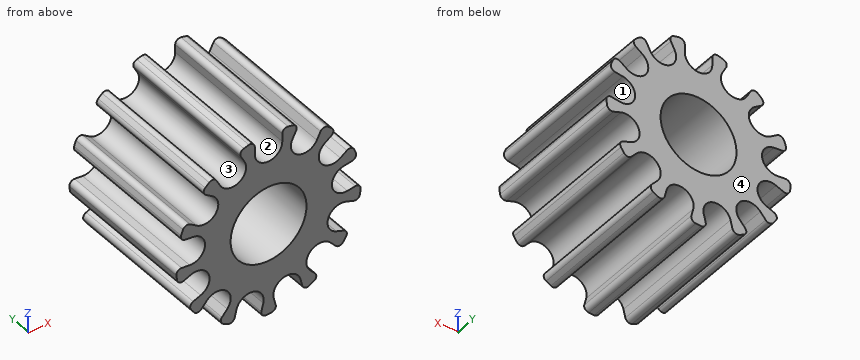
from build123d import *

# Parameters (mm, degrees)
BOSS_EXTRUDE1_DEPTH      = 7.5
CUT_EXTRUDE1_START       = -7.5
CUT_EXTRUDE1_DEPTH       = 15
FILLET1_R                = 0.5
CIRPATTERN1_COUNT        = 13
FILLET1_OF_CIRPATTERN1_R = 0.5
CUT_EXTRUDE2_DEPTH       = 16.666124697
CUT_EXTRUDE2_DEPTH_BACK  = 16.666124697
SKETCH7_R                = 4


# Read off the part's stored shape, not the designer's step: Cut-Extrude1
with BuildPart() as part:
    # Sketch5 → Boss-Extrude1 (new, symmetric)
    with BuildSketch(Plane(origin=(0, 0, 0), x_dir=(1, 0, 0), z_dir=(0, 1, 0))):
        with BuildLine():
            ThreePointArc((-0.898321896, 9.703578331), (-2.332148212, 9.46189724), (-3.714053167, 9.009562905))
            Line((-3.714053167, 9.009562905), (-3.369074568, 7.60992971))
            ThreePointArc((-3.369074568, 7.60992971), (-1.614201219, 6.549071788), (-0.553343297, 8.303945136))
            Line((-0.553343297, 8.303945136), (-0.898321896, 9.703578331))
        make_face()
        with BuildLine():
            Line((-3.369074568, 7.60992971), (-3.714053167, 9.009562905))
            ThreePointArc((-3.714053167, 9.009562905), (-5.420917899, -8.098151875), (9.745071301, 0))
            ThreePointArc((9.745071301, 0), (6.565523731, 7.201410473), (-0.898321896, 9.703578331))
            Line((-0.898321896, 9.703578331), (-0.553343297, 8.303945136))
            ThreePointArc((-0.553343297, 8.303945136), (-1.614201219, 6.549071788), (-3.369074568, 7.60992971))
        make_face()
    extrude(amount=BOSS_EXTRUDE1_DEPTH, both=True)

    # Cut-Extrude1 outline → Cut-Extrude1 (cut)
    with BuildSketch(Plane(origin=(0, 0, 0), x_dir=(1, 0, 0), z_dir=(0, 1, 0)).offset(CUT_EXTRUDE1_START)):
        with BuildLine():
            ThreePointArc((-0.898321896, 9.703578331), (-2.332148212, 9.46189724), (-3.714053167, 9.009562905))
            Line((-3.714053167, 9.009562905), (-3.369074568, 7.60992971))
            ThreePointArc((-3.369074568, 7.60992971), (-1.61420122, 6.549071788), (-0.553343297, 8.303945136))
            Line((-0.553343297, 8.303945136), (-0.898321896, 9.703578331))
        make_face()
    cut_extrude1 = extrude(amount=CUT_EXTRUDE1_DEPTH, mode=Mode.SUBTRACT)

    # Fillet1
    fillet1_edges = [part.edges().sort_by_distance(p)[0] for p in [
        (-3.714053167, 0, -9.009562905),
        (-0.898321896, 0, -9.703578331),
    ]]
    fillet(fillet1_edges, radius=FILLET1_R)

    # CirPattern1: Cut-Extrude1 ×13 about axis
    cirpattern1_axis = Axis((0, 0, 0), (0, 1, 0))
    for i in range(1, CIRPATTERN1_COUNT):
        add(cut_extrude1.rotate(cirpattern1_axis, i * 360 / CIRPATTERN1_COUNT), mode=Mode.SUBTRACT)

    # Fillet1 of CirPattern1
    fillet1_of_cirpattern1_edges = [part.edges().sort_by_distance(p)[0] for p in [
        (-7.475583408, 0, -6.251565194),
        (-5.304902238, 0, -8.174620903),
        (-9.524547581, 0, -2.061409236),
        (-8.496193408, 0, -4.77295634),
        (-9.391552687, 0, 2.600990735),
        (-9.741109059, 0, -0.277865001),
        (-7.107066252, 0, 6.667535074),
        (-8.754454018, 0, 4.280881862),
        (-3.194436588, 0, 9.20662748),
        (-5.762259063, 0, 7.85893028),
        (1.45, 0, 9.636592482),
        (-1.45, 0, 9.636592482),
        (5.762259064, 0, 7.85893028),
        (3.194436589, 0, 9.206627479),
        (8.754454018, 0, 4.280881862),
        (7.107066252, 0, 6.667535073),
        (9.741109059, 0, -0.277865001),
        (9.391552686, 0, 2.600990734),
        (8.496193408, 0, -4.772956341),
        (9.524547581, 0, -2.061409237),
        (5.304902238, 0, -8.174620903),
        (7.475583408, 0, -6.251565194),
        (0.898321896, 0, -9.703578332),
        (3.714053167, 0, -9.009562905),
    ]]
    fillet(fillet1_of_cirpattern1_edges, radius=FILLET1_OF_CIRPATTERN1_R)

    # Sketch7 → Cut-Extrude2 (cut, two sides: drawn at the far end of the back side and taken through both)
    with BuildSketch(Plane(origin=(0, 0, 0), x_dir=(1, 0, 0), z_dir=(0, 1, 0)).offset(-CUT_EXTRUDE2_DEPTH_BACK)):
        with Locations(Location((0, 0, 0), (0, 0, 270))):
            Circle(SKETCH7_R)
    extrude(amount=CUT_EXTRUDE2_DEPTH + CUT_EXTRUDE2_DEPTH_BACK, mode=Mode.SUBTRACT)


solid = part.part
The model under review builds one solid part; all positions refer to its coordinate system, in mm. Face numbers are marked on the shaded views. A direction names the side the tool comes from. Coordinates: 2 decimals unless noted, no trailing zeros. Write each loop counter-clockwise with the first axis right and the second up, starting at its lowest first coordinate (ties: lowest second). Pieces come first, ordered by that corner, then holes. Notation, with made-up numbers: (26, -30.5) -> (62, -30.5) arc R14 cw to (62, -23.5) -> close; hole circle Ø6 at (40.25, 62.25). An arc over 180 degrees is marked (long way). Answer in a Markdown table with one row per item.
1. Draft analysis for pull direction X (two halves, no side actions). For the marked faces 3 and 4, state which applies: +X half, -X half, draft (parallel to the pull), parting line (faces both ways), or undercut.
Answers below:
| item | result |
|---|---|
| face 3 | undercut |
| face 4 | draft |
2. For the marked faces 1 and 2, list the 3-axis set-ups (+Z, -Z, +X, -X, +Y, -Y) from which the entire face can be reached by the end or side of a thin tool; tool diameter is ignored.
Answers below:
| item | result |
|---|---|
| face 1 | +Y, -Y |
| face 2 | +Z, +Y, -Y |
3. Wall thickness on probe 1 along X at (y, z) = (0, 0); probe 2 along Z at (x, y) = (0, -0.5); probe 3 along X at (y, z) = (6.5, 6): over which ranges is each line inside the solid? List them lowest first. Write a range as [from, to].
Answers below:
| item | result |
|---|---|
| probe 1 | x = [-7.07, -4], [4, 7.07] |
| probe 2 | z = [-9.75, -4], [4, 6.75] |
| probe 3 | x = [-6.14, -4.53], [-3.08, 3.08], [4.53, 6.14] |
4. We need section A-A, the plane x = 0. State the section outline as (y, z) points, and give its area (3 significant figures).
Answers below:
| item | result |
|---|---|
| outline | (-7.5, -9.75) -> (7.5, -9.75) -> (7.5, -4) -> (-7.5, -4) -> close; (-7.5, 4) -> (7.5, 4) -> (7.5, 6.75) -> (-7.5, 6.75) -> close |
| area | 127 mm^2 |
5. Clearance check with flat-ended pins moving along their axes: pin 1 Ø1 at (y, z) = (2.5, 4) entering from -X; pin 2 Ø5 at (x, z) = (0, 0) entering from -Y; pin 3 Ø1.5 at (x, y) = (-6.5, 2.5) entering from +Z. State where each tip first meets the part, or that it passes through.
Answers below:
| item | result |
|---|---|
| pin 1 | stops at x = -9.09 |
| pin 2 | passes through |
| pin 3 | stops at z = 7.6 |
6. We need section B-B, the plane z = -3. State the section outline as (x, y) points.
Answers below:
| item | result |
|---|---|
| outline | (-6.22, -7.5) -> (-2.65, -7.5) -> (-2.65, 7.5) -> (-6.22, 7.5) -> close; (2.65, -7.5) -> (6.22, -7.5) -> (6.22, 7.5) -> (2.65, 7.5) -> close |
